Geometry: final body of the model. Coordinates: model frame, mm. A direction names the side the tool comes from. Round coordinates to 2 decimals unless told otherwise and drop trailing zeros. Loops run counter-clockwise (first coordinate to the right, second up) from the corner with the lowest first, then second, coordinate; pieces in that order, holes last. Notation, with made-up numbers: (9.25, -2.75) -> (29.25, -2.75) arc R27 ccw to (29.25, 28.25) -> close; hole circle Ø8 at (40, -40). An arc over 180 degrees is marked (long way). Answer in a Markdown table with one row per item.
```python
from build123d import *

# Parameters (mm, degrees)
SKETCH1_W           = 11.112
SKETCH1_H           = 15.43
SKETCH1_W_2         = 7.112
SKETCH1_H_2         = 11.43
BOSS_EXTRUDE1_DEPTH = 203.2
SKETCH2_W           = 11.112
SKETCH2_H           = 25.59
SKETCH2_W_2         = 7.112
SKETCH2_H_2         = 11.43
BOSS_EXTRUDE2_DEPTH = 3.175


with BuildPart() as part:
    # Sketch1 → Boss-Extrude1 (new body)
    with BuildSketch(Plane(origin=(0, 0, 0), x_dir=(1, 0, 0), z_dir=(0, 1, 0))):
        with Locations((5.556, 7.715)):
            Rectangle(SKETCH1_W, SKETCH1_H)
        with Locations((5.556, 7.715)):
            Rectangle(SKETCH1_W_2, SKETCH1_H_2, mode=Mode.SUBTRACT)
    extrude(amount=BOSS_EXTRUDE1_DEPTH)

    # Sketch2 → Boss-Extrude2 (add)
    with BuildSketch(Plane.XZ):
        with Locations((5.556, -12.795)):
            Rectangle(SKETCH2_W, SKETCH2_H)
        with Locations((5.556, -7.715)):
            Rectangle(SKETCH2_W_2, SKETCH2_H_2, mode=Mode.SUBTRACT)
    extrude(amount=BOSS_EXTRUDE2_DEPTH)


solid = part.part
```
Item 1: Section query A-A, the plane x = 5.5. Output: boundary loops of the cut face in (y, z) (3 decimals), and give its area (3 significant figures).
Ans:
| item | result |
|---|---|
| outline | (-3.175, -25.59) -> (0, -25.59) -> (0, -15.43) -> (203.2, -15.43) -> (203.2, -13.43) -> (-3.175, -13.43) -> close; (-3.175, -2) -> (203.2, -2) -> (203.2, 0) -> (-3.175, 0) -> close |
| area | 858 mm2 |
Item 2: Mould query, pull axis Z, two halves, no side actions, for faces 4 (the flat face through (1.8, 203.2, -7.8)), 5 (the flat face through (5, -2, -25.59)), 6 (the flat face through (6, 101, -13.43)), 7 (the flat face through (5, 101, 0)). Classes: released by +Z, released by -Z, zero draft, split by the parting line, or undercut.
Ans:
| item | result |
|---|---|
| face 4 | zero draft |
| face 5 | released by -Z |
| face 6 | undercut |
| face 7 | released by +Z |
Item 3: Section query B-B, the plane y = 94. Output: boundary loops of the cut face in (x, z).
Ans:
| item | result |
|---|---|
| outline | (0, -15.43) -> (11.11, -15.43) -> (11.11, 0) -> (0, 0) -> close; hole (2, -13.43) -> (9.11, -13.43) -> (9.11, -2) -> (2, -2) -> close |
Item 4: Set-up query: faces 1 (the flat face through (11.112, 101, -7)), 2 (the flat face through (5, 0, -20)), 3 (the flat face through (2, 101, -8)). Return all of +Z, -Z, +X, -X, +Y, -Y with unobstructed straight access to the full face (end or side cutting, diameter ignored); none if empty.
Ans:
| item | result |
|---|---|
| face 1 | +Z, -Z, +X, +Y, -Y |
| face 2 | -Z, +X, -X, +Y |
| face 3 | +Y, -Y |
Item 5: Ray query, L1, parallel to X at y = 169.5, z = -11.5; L2, parallel to Z at x = 4.25, y = 76; L3, parallel to Y at x = 10.5, z = -15.75 (3 decimals). Return the intervals inside material, ascending.
Ans:
| item | result |
|---|---|
| L1 | 0 to 2, 9.11 to 11.11 |
| L2 | -15.43 to -13.43, -2 to 0 |
| L3 | -3.175 to 0 |
Item 6: First-contact query: P1, Ø2, axis at y = 53, z = -16, coming from the -X side; P2, Ø3, axis at x = 1.5, y = 146.5, coming from the -Z side. Flat tips, straight axial feed; report the tip coordinate or a pass-through.
Ans:
| item | result |
|---|---|
| P1 | x = 0 |
| P2 | z = -15.43 |
